Can you work these out from the drawing? Everything is in mm from the part's minimum corner. A direction names the side the tool comes from. Round coordinates to 2 decimals unless told otherwise and drop trailing zeros. Write each loop counter-clockwise with the first axis right and the second up, starting at its lowest first coordinate (ties: lowest second). Pieces come first, ordered by that corner, then holes. Notation, with made-up numbers: (10, 28) - (66, 28) arc R23 ccw to (66, 54) - close; hole circle Ø11 at (79, 1.25). An arc over 180 degrees is marked (long way). One line per item, written item: value. Start each with the question number.
Item 1: If I drill on line 1 (Z direction, x = 19.05, y = 15); line 2 (X direction, y = 19, z = 62) (1 decimal); line 3 (Z direction, x = 9, y = 13), over which ranges is the centre line in solid material (lowest first)?
Item 2: Imagine slicing it at C-C, the plane z = 23. Please give me the cut outline in (x, y) (3 decimals).
Item 3: For P1, Ø4, axis at y = 27.5, z = 59.5, coming from the +X side; P2, Ø7.5, axis at x = 19.05, z = 62.23, coming from the -Y side (3 decimals); P3, Ø3, axis at y = 26, z = 19, coming from the +X side, each with a flat end and sliding along its axis, tell me the tip position at first contact or that it passes through.
Item 4: For the marked faces 1 and 2, which set-ups out of +Z, -Z, +X, -X, +Y, -Y let a thin tool reach every point of the face, with its end or its side?
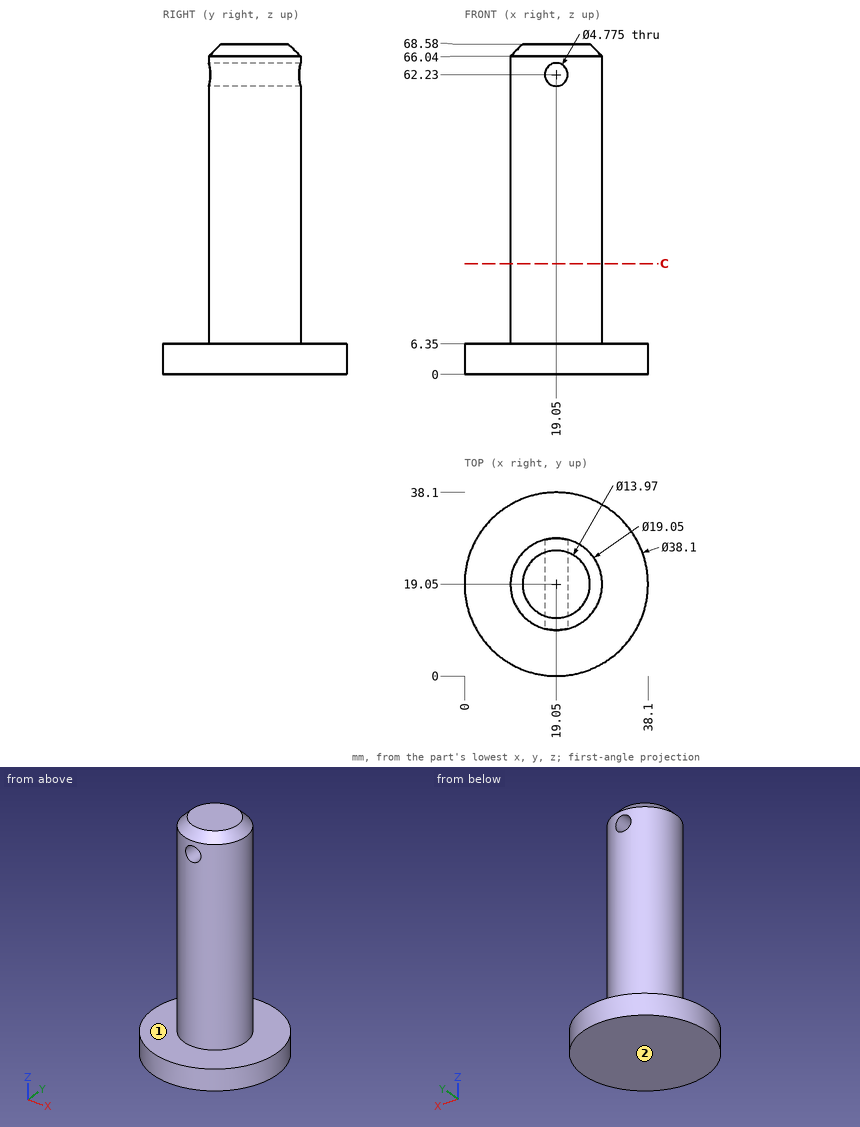
Values follow:
1. line 1: z = 0 to 59.84, 64.62 to 68.58
1. line 2: x = 9.5 to 16.7, 21.4 to 28.6
1. line 3: z = 0 to 6.35
2. outline: circle Ø19.05 at (19.05, 19.05)
3. P1: stops at x = 26.06
3. P2: stops at y = 9.525
3. P3: stops at x = 26.86
4. face 1: +Z
4. face 2: -Z, +X, -X, +Y, -Y
